The listing builds one solid part. Answer for the finished solid, in the listing's coordinates (mm). A direction names the side the tool comes from. Coordinates: 2 decimals unless noted, no trailing zeros. Loops run counter-clockwise (first coordinate to the right, second up) from the corner with the lowest first, then second, coordinate; pieces in that order, holes last. Notation, with made-up numbers: (73, 61.5) - (87, 61.5) arc R9 cw to (87, 68.5) - close; hole circle Ø5 at (1, -20). An arc over 180 degrees is marked (long way). Put each result on its own line as item: value.
```python
from build123d import *

# Parameters (mm, degrees)
DODANIE_WYCI_GNI_CIE1_DEPTH = 9
SZKIC3_R                    = 17.5
SZKIC3_R_2                  = 7
DODANIE_WYCI_GNI_CIE2_DEPTH = 9
DODANIE_WYCI_GNI_CIE3_START = -9
SZKIC4_R                    = 17.5
SZKIC4_R_2                  = 7
DODANIE_WYCI_GNI_CIE3_DEPTH = 9


with BuildPart() as part:
    # Szkic1 → Dodanie-wyciągnięcie1 (new body)
    with BuildSketch(Plane.XY):
        with BuildLine():
            Line((0, 20), (-86, 20))
            Line((-86, 20), (-86, -20))
            Line((-86, -20), (0, -20))
            ThreePointArc((0, -20), (20, 0), (0, 20))
        make_face()
        with BuildLine():
            ThreePointArc((-23, -7), (-30, 0), (-23, 7))
            Line((-23, 7), (0, 7))
            ThreePointArc((0, 7), (4.949747468, 4.949747468), (7, 0))
            ThreePointArc((7, 0), (4.949747468, -4.949747468), (0, -7))
            Line((0, -7), (-23, -7))
        make_face(mode=Mode.SUBTRACT)
    extrude(amount=DODANIE_WYCI_GNI_CIE1_DEPTH)

    # Szkic3 → Dodanie-wyciągnięcie2 (add)
    # profile 1 of 2: a face of its own
    with BuildSketch(Plane.XZ.offset(20)):
        with Locations((-68.5, 35)):
            Circle(SZKIC3_R)
        with Locations((-68.5, 35)):
            Circle(SZKIC3_R_2, mode=Mode.SUBTRACT)
    # profile 2 of 2: a face of its own
    with BuildSketch(Plane.XZ.offset(20)):
        with BuildLine():
            Line((-86, 35), (-86, 9))
            Line((-86, 9), (-51, 9))
            Line((-51, 9), (-51, 35))
            ThreePointArc((-51, 35), (-68.5, 17.5), (-86, 35))
        make_face()
    extrude(amount=-DODANIE_WYCI_GNI_CIE2_DEPTH)

    # Szkic4 → Dodanie-wyciągnięcie3 (add)
    # profile 1 of 2: a face of its own
    with BuildSketch(Plane(origin=(0, 20, 0), x_dir=(1, 0, 0), z_dir=(0, 1, 0)).offset(DODANIE_WYCI_GNI_CIE3_START)):
        with BuildLine():
            Line((-51, -9), (-86, -9))
            Line((-86, -9), (-86, -35))
            ThreePointArc((-86, -35), (-68.5, -17.5), (-51, -35))
            Line((-51, -35), (-51, -9))
        make_face()
    # profile 2 of 2: a face of its own
    with BuildSketch(Plane(origin=(0, 20, 0), x_dir=(1, 0, 0), z_dir=(0, 1, 0)).offset(DODANIE_WYCI_GNI_CIE3_START)):
        with Locations((-68.5, -35)):
            Circle(SZKIC4_R)
        with Locations((-68.5, -35)):
            Circle(SZKIC4_R_2, mode=Mode.SUBTRACT)
    extrude(amount=DODANIE_WYCI_GNI_CIE3_DEPTH)


solid = part.part
```
1) The part is cut by section A-A (x = -6.5). Give the vertices of the cut face in (y, z).
Found:
outline: (-20, 0) - (-7, 0) - (-7, 9) - (-20, 9) - close; (7, 0) - (20, 0) - (20, 9) - (7, 9) - close
2) The part is cut by section D-D (y = -4.5). Give the vertices of the cut face in (x, z), and give its area (3 significant figures).
Found:
outline: (-86, 0) - (-28.36, 0) - (-28.36, 9) - (-86, 9) - close; (5.36, 0) - (19.49, 0) - (19.49, 9) - (5.36, 9) - close
area: 646 mm^2
3) For faces 5 (the face through (-51, -16, 22)), 6 (the face through (-30, 0, 4)), 7 (the face through (-69, -11, 26)), determine the directions among +Z, -Z, +X, -X, +Y, -Y from which every point of the face is accessible in a straight line to the end or side of a thin tool.
Found:
face 5: +Z, +X, +Y, -Y
face 6: +Z, -Z
face 7: +Z, +X, -X
4) Each of these flat-tipped pins is pushed along its axis until it touches: pin 1 (8 mm diameter, centred on x = -34, y = 9.5, fed in from +Z); pin 2 (3 mm diameter, centred on x = -72.5, y = -11.5, fed in from +Z); pin 3 (11 mm diameter, centred on x = -68.5, z = 35, fed in from -Y); pin 4 (2.5 mm diameter, centred on y = 16, z = 17, fed in from +X). Where does it stop, or does it pass through?
Found:
pin 1: stops at z = 9
pin 2: stops at z = 52.32
pin 3: passes through
pin 4: stops at x = -51
5) The part is cut by section C-C (z = 4.5). Give the vertices of the cut face in (x, y).
Found:
outline: (-86, -20) - (0, -20) arc R20 ccw to (0, 20) - (-86, 20) - close; hole (-23, -7) - (0, -7) arc R7 ccw to (0, 7) - (-23, 7) arc R7 ccw to start
6) For a pull along X with two mould halves and no side action, classify faces 1 (the face through (-12, 7, 4)), 2 (the face through (-68.885, 15.437, 52.496)), 3 (the face through (-69, 11, 26)), 4 (the face through (-11, -7, 4)) as pulls with the +X half, pulls with the -X half, needs draft (parallel to the pull), parting line crosses it, or undercut.
Found:
face 1: undercut
face 2: parting line crosses it
face 3: needs draft
face 4: undercut
7) The part is cut by section B-B (x = -68.5). Give the vertices of the cut face in (y, z), and give its area (3 significant figures).
Found:
outline: (-20, 0) - (20, 0) - (20, 28) - (11, 28) - (11, 9) - (-11, 9) - (-11, 28) - (-20, 28) - close; (-20, 42) - (-11, 42) - (-11, 52.5) - (-20, 52.5) - close; (11, 42) - (20, 42) - (20, 52.5) - (11, 52.5) - close
area: 891 mm^2
8) Straight lines are drawn through the part: L1, parallel to Y at x = -71.5, z = 12; L2, parallel to Z at x = -68, y = -14; L3, parallel to X at y = 17.75, z = 35. For each, find the intervals that lie inside material, in ascending order. Write a range as [from, to].
Found:
L1: y = [-20, -11], [11, 20]
L2: z = [0, 28.02], [41.98, 52.49]
L3: x = [-86, -75.5], [-61.5, -51]
